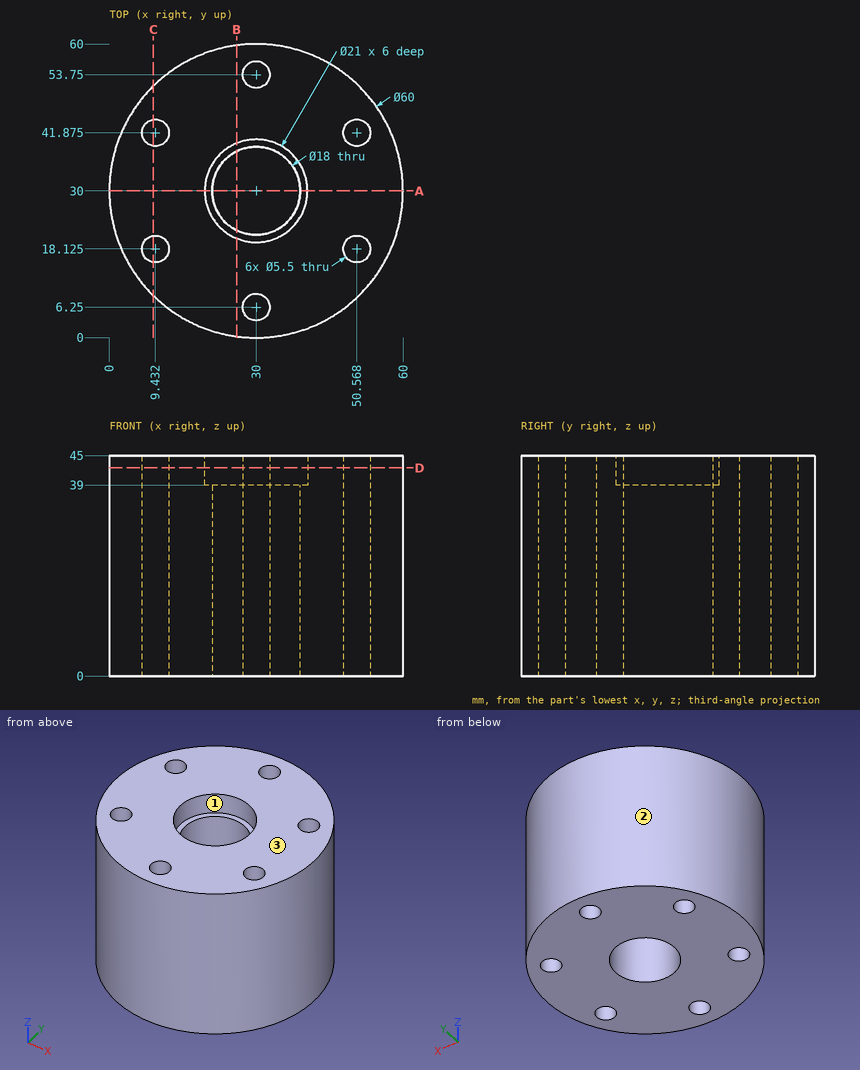
Design review of the part shown in the three views and the two pictorial views. Dimensions are in mm from the part's minimum x, y and z. Round coordinates to 2 decimals unless told otherwise and drop trailing zeros. Write each loop counter-clockwise with the first axis right and the second up, starting at its lowest first coordinate (ties: lowest second). Pieces come first, ordered by that corner, then holes.
Item 1: Consider section B-B on x = 26. Give the boundary of the cut face in (y, z).
Item 2: Consider section C-C on x = 9. Give the boundary of the cut face in (y, z), and give its area (3 significant figures).
Item 3: Wall thickness on L1, parallel to Y at x = 30, z = 27; L2, parallel to X at y = 16, z = 30.5; L3, parallel to X at y = 6, z = 35: over which ranges is each line inside the solid? List them lowest first.
Item 4: Consider section A-A on y = 30. Give the boundary of the cut face in (x, z), and give its area (3 significant figures).
Item 5: Consider section D-D on z = 42.5. Give the boundary of the cut face in (x, y) (3 decimals), and give its area (3 significant figures).
Item 6: Draft analysis for pull direction Y (two halves, no side actions). For the marked faces 1, 2 and 3, state which applies: released by +Y, released by -Y, zero draft, split by the parting line, or undercut.
Item 7: For pin 1 Ø4 at (y, z) = (10, 10) entering from -X; pin 2 Ø4 at (y, z) = (23, 19.5) entering from -X; pin 3 Ø1 at (y, z) = (18, 13.5) entering from -X, all flat-tipped, find the tip position at first contact; note any pin that passes through.
Check values:
1. outline: (0.27, 0) - (21.94, 0) - (21.94, 39) - (20.29, 39) - (20.29, 45) - (0.27, 45) - close; (38.06, 0) - (59.73, 0) - (59.73, 45) - (39.71, 45) - (39.71, 39) - (38.06, 39) - close
2. outline: (8.58, 0) - (15.41, 0) - (15.41, 45) - (8.58, 45) - close; (20.84, 0) - (39.16, 0) - (39.16, 45) - (20.84, 45) - close; (44.59, 0) - (51.42, 0) - (51.42, 45) - (44.59, 45) - close
2. area: 1,440 mm2
3. L1: y = 0 to 3.5, 9 to 21, 39 to 51, 56.5 to 60
3. L2: x = 3.47 to 7.69, 11.18 to 48.82, 52.31 to 56.53
3. L3: x = 12 to 27.26, 32.74 to 48
4. outline: (0, 0) - (21, 0) - (21, 39) - (19.5, 39) - (19.5, 45) - (0, 45) - close; (39, 0) - (60, 0) - (60, 45) - (40.5, 45) - (40.5, 39) - (39, 39) - close
4. area: 1,870 mm2
5. outline: circle Ø60 at (30, 30); hole circle Ø5.5 at (9.432, 18.125); hole circle Ø5.5 at (9.432, 41.875); hole circle Ø21 at (30, 30); hole circle Ø5.5 at (30, 6.25); hole circle Ø5.5 at (30, 53.75); hole circle Ø5.5 at (50.568, 18.125); hole circle Ø5.5 at (50.568, 41.875)
5. area: 2,340 mm2
6. face 1: undercut
6. face 2: split by the parting line
6. face 3: zero draft
7. pin 1: stops at x = 6
7. pin 2: stops at x = 0.42
7. pin 3: stops at x = 2.29
